Read the model definition and answer for the solid it produces. Units are mm, in the model's axes. A direction names the side the tool comes from. Round coordinates to 2 decimals unless told otherwise and drop trailing zeros. Order: outer loops, then holes, each group sorted by start corner. A loop starts at its lowest first (then second) coordinate and runs counter-clockwise, first axis right, second up.
from build123d import *

# Parameters (mm, degrees)
SKETCH_1_W          = 180
SKETCH_1_H          = 145
EXTRUDE_1_DEPTH     = 1.5
SKETCH_2_R          = 2.1
SKETCH_2_W          = 53
SKETCH_2_H          = 92
CUT_EXTRUDE_1_DEPTH = 116.608174451
SKETCH_4_W          = 18
SKETCH_4_H          = 32
CUT_EXTRUDE_3_DEPTH = 116.608174451
SKETCH_3_R          = 1
CUT_EXTRUDE_2_DEPTH = 116.608174451
FILLET_1_R          = 2.5
CHAMFER_1_SIZE      = 2
CHAMFER_2_SIZE      = 10
CHAMFER_3_SIZE      = 4
SKETCH_5_R          = 1.35
SKETCH_5_W          = 32
SKETCH_5_H          = 71
CUT_EXTRUDE_4_DEPTH = 116.608174451
FILLET_2_R          = 1


with BuildPart() as part:
    # 草图1 → 凸台-拉伸1 (new, symmetric)
    with BuildSketch(Plane.XY):
        Rectangle(SKETCH_1_W, SKETCH_1_H)
    extrude(amount=EXTRUDE_1_DEPTH, both=True)

    # 草图2 → 切除-拉伸1 (cut, through all)
    with BuildSketch(Plane.XY.offset(1.5)):
        with Locations((-70, 62.5)):
            Circle(SKETCH_2_R)
        with Locations((-70, -62.5)):
            Circle(SKETCH_2_R)
        with Locations((70, -62.5)):
            Circle(SKETCH_2_R)
        with Locations((70, 62.5)):
            Circle(SKETCH_2_R)
        with Locations((63.5, 0)):
            Rectangle(SKETCH_2_W, SKETCH_2_H)
    extrude(amount=-CUT_EXTRUDE_1_DEPTH, mode=Mode.SUBTRACT)

    # 草图4 → 切除-拉伸3 (cut, through all)
    with BuildSketch(Plane.XY.offset(1.5)):
        with Locations((28, -3.5)):
            Rectangle(SKETCH_4_W, SKETCH_4_H)
    extrude(amount=-CUT_EXTRUDE_3_DEPTH, mode=Mode.SUBTRACT)

    # 草图3 → 切除-拉伸2 (cut, through all)
    with BuildSketch(Plane.XY.offset(1.5)):
        with Locations((38, 46)):
            Circle(SKETCH_3_R)
        with Locations((38, -46)):
            Circle(SKETCH_3_R)
    extrude(amount=-CUT_EXTRUDE_2_DEPTH, mode=Mode.SUBTRACT)

    # 圆角1
    fillet_1_edges = [part.edges().sort_by_distance(p)[0] for p in [
        (19, -19.5, 0),
        (19, 12.5, 0),
    ]]
    fillet(fillet_1_edges, radius=FILLET_1_R)

    # 倒角1
    chamfer_1_edges = [part.edges().sort_by_distance(p)[0] for p in [
        (67.9, 62.5, -1.5),
        (67.9, -62.5, -1.5),
        (-72.1, -62.5, -1.5),
        (-72.1, 62.5, -1.5),
    ]]
    chamfer(chamfer_1_edges, length=CHAMFER_1_SIZE)

    # 倒角2
    chamfer_2_edges = [part.edges().sort_by_distance(p)[0] for p in [
        (-90, 72.5, 0),
        (90, 72.5, 0),
        (90, -72.5, 0),
        (-90, -72.5, 0),
    ]]
    chamfer(chamfer_2_edges, length=CHAMFER_2_SIZE)

    # 倒角3
    chamfer_3_edges = [part.edges().sort_by_distance(p)[0] for p in [
        (90, 46, 0),
        (90, -46, 0),
        (37, 12.5, 0),
        (37, -19.5, 0),
    ]]
    chamfer(chamfer_3_edges, length=CHAMFER_3_SIZE)

    # 草图5 → 切除-拉伸4 (cut, through all)
    with BuildSketch(Plane.XY.offset(1.5)):
        with Locations((-71, 44.5)):
            Circle(SKETCH_5_R)
        with Locations((-29, 44.5)):
            Circle(SKETCH_5_R)
        with Locations((-71, -18.5)):
            Circle(SKETCH_5_R)
        with Locations((-29, -18.5)):
            Circle(SKETCH_5_R)
        with Locations((-50, 12)):
            Rectangle(SKETCH_5_W, SKETCH_5_H)
    extrude(amount=-CUT_EXTRUDE_4_DEPTH, mode=Mode.SUBTRACT)

    # 圆角2
    fillet_2_edges = [part.edges().sort_by_distance(p)[0] for p in [
        (-66, -23.5, 0),
        (-66, 47.5, 0),
        (-34, 47.5, 0),
        (-34, -23.5, 0),
    ]]
    fillet(fillet_2_edges, radius=FILLET_2_R)


solid = part.part
Q1. A cutting plane is placed at C-C, the plane x = 70. Give the vertices of the cut face in (y, z), plus the area to 3 significant figures.
Outcome:
outline: (-72.5, -1.5) - (-66.6, -1.5) - (-64.6, 0.5) - (-64.6, 1.5) - (-72.5, 1.5) - close; (-60.4, 0.5) - (-58.4, -1.5) - (-46, -1.5) - (-46, 1.5) - (-60.4, 1.5) - close; (46, -1.5) - (58.4, -1.5) - (60.4, 0.5) - (60.4, 1.5) - (46, 1.5) - close; (64.6, 0.5) - (66.6, -1.5) - (72.5, -1.5) - (72.5, 1.5) - (64.6, 1.5) - close
area: 126 mm2
Q2. For faces 4 (the face through (69.54, 60.45, 1.01)), 5 (the face through (35, -21.5, 0)), determine the directions among +Z, -Z, +X, -X, +Y, -Y from which every point of the face is accessible in a straight line to the end or side of a thin tool.
Outcome:
face 4: +Z, -Z
face 5: +Z, -Z, +X
Q3. A cutting plane is placed at B-B, the plane y = 36. Give the vertices of the cut face in (x, z), plus the area to 3 significant figures.
Outcome:
outline: (-90, -1.5) - (-66, -1.5) - (-66, 1.5) - (-90, 1.5) - close; (-34, -1.5) - (37, -1.5) - (37, 1.5) - (-34, 1.5) - close
area: 285 mm2
Q4. A cutting plane is placed at D-D, the plane z = -0.7. Give the number of separate pieces and of enclosed holes in the cut face, plus the area to 3 significant figures.
Outcome:
separate pieces: 1
enclosed holes: 9
area: 18,000 mm2
Q5. For a pull along Y with two mould halves and no side action, classify faces 1 (the face through (88, -48, 0)), 2 (the face through (-84.9, -67.6, 0)), 3 (the face through (-1, 1, -1.5)) as released by +Y, released by -Y, zero draft, split by the parting line, or undercut.
Outcome:
face 1: undercut
face 2: released by -Y
face 3: zero draft
Q6. A cutting plane is placed at A-A, the plane x = -40. Give the vertices of the cut face in (y, z).
Outcome:
outline: (-72.5, -1.5) - (-23.5, -1.5) - (-23.5, 1.5) - (-72.5, 1.5) - close; (47.5, -1.5) - (72.5, -1.5) - (72.5, 1.5) - (47.5, 1.5) - close
Q7. Flat-ended cylindrical pins translate along their axes: pin 1 (0.9 mm diameter, centred on y = -31.5, z = 0.5, fed in from +X); pin 2 (6.5 mm diameter, centred on x = 70, y = 62.5, fed in from -Z). Find the tip coordinate at first contact, or state that the pin passes through.
Outcome:
pin 1: stops at x = 37
pin 2: stops at z = -0.65
Q8. Straight lines are drawn through the part: probe 1 along Y at (x, z) = (70, 1.05); probe 2 along X at (y, z) = (-15, -1.1); probe 3 along X at (y, z) = (41, 1.1). For each, find the intervals that lie inside material, in ascending order.
Outcome:
probe 1: y = -72.5 to -64.6, -60.4 to -46, 46 to 60.4, 64.6 to 72.5
probe 2: x = -90 to -66, -34 to 19
probe 3: x = -90 to -66, -34 to 37
